Verification items for the finished model (mm, model axes). A direction names the side the tool comes from. Give positions to 0.01 mm unless a question says otherwise; leave off trailing zeros. Write each loop counter-clockwise with the first axis right and the second up, starting at its lowest first coordinate (ties: lowest second). Pieces come first, ordered by that corner, then holes. Notation, with made-up numbers: (-19, -24) - (40, -24) arc R29 cw to (40, 10) - close; hole circle Ø8 at (67.25, 19.25). An arc over 180 degrees is marked (long way). Answer as a JSON object with one key per item and string values. Group by question number.
Item 1: Go/stop test with flat-tipped pins: pin 1 (12 mm diameter, centred on x = -45, y = -17, fed in from +Z); pin 2 (6 mm diameter, centred on x = -51, y = -14.5, fed in from -Z). Record where each tip stops, or that it passes through.
Item 2: Scan lines: line 1 along X through (y, z) = (-7.5, 26); line 2 along Z through (x, y) = (-38, -12.75); line 3 along Z through (x, y) = (-54.5, -3.75). Record each from-to range of solid material in increasing order. Write a range as [from, to].
Item 3: Draft check along X on faces 4 (the face through (-61.296, -13, 18)), 5 (the face through (-43, -13, 0)), 6 (the face through (-48.884, -13, 27)). Enter one of: +X half, -X half, draft (parallel to the pull), parting line (faces both ways), or undercut.
Item 4: Sectioned sample at B-B, the plane y = -15.75. Record the boundary of the cut face in (x, z).
Item 5: Sectioned sample at A-A, the plane z = 20. Record the boundary of the cut face in (x, y).
Item 6: Tool access check on faces 1 (the face through (-37.809, -13, 27)), 2 (the face through (-55, -13, 34.945)), 3 (the face through (-43, 0, 18)). Record the directions out of +Z, -Z, +X, -X, +Y, -Y that give a thin tool (end or side, any length) a straight path to the whole face; none if there is none.
```python
from build123d import *

# Parameters (mm, degrees)
F1_DEPTH = 25.4
F4_DEPTH = 25.4


with BuildPart() as f1:
    # F0 (on Front) → F1 (new body)
    with BuildSketch(Plane.XZ):
        Polygon((-51.1758476496, 56.7135326564), (-63.5878965259, 56.522578001), (-63.5878965259, 0), (-8.4020039067, 0), (-8.4020039067, 56.522578001), (-21.959785372, 56.522578001), (-21.959785372, 11.6482349113), (-51.1758476496, 11.6482349113), align=None)
    extrude(amount=F1_DEPTH)


with BuildPart() as f4:
    # F3 (on Front) → F4 (new body)
    with BuildSketch(Plane.XZ):
        Polygon((-61.2964443862, 34.9447019398), (-61.2964443862, 33.4170646966), (-61.2964443862, 0), (-24.4421958923, 0), (-24.4421958923, 35.1356565952), (-37.809021771, 35.1356565952), (-37.809021771, 19.2864201963), (-48.8843917847, 19.2864201963), (-48.8843917847, 34.9447019398), align=None)
    extrude(amount=F4_DEPTH)


solid = f4.part
```
Geometry check:
{
 "1": {"pin 1": "z = 34.94", "pin 2": "z = 0"},
 "2": {"line 1": "[-61.3, -48.88], [-37.81, -24.44]", "line 2": "[0, 19.29]", "line 3": "[0, 34.94]"},
 "3": {"face 4": "-X half", "face 5": "draft", "face 6": "undercut"},
 "4": {"outline": "(-61.3, 0) - (-24.44, 0) - (-24.44, 35.14) - (-37.81, 35.14) - (-37.81, 19.29) - (-48.88, 19.29) - (-48.88, 34.94) - (-61.3, 34.94) - close"},
 "5": {"outline": "(-61.3, -25.4) - (-48.88, -25.4) - (-48.88, 0) - (-61.3, 0) - close; (-37.81, -25.4) - (-24.44, -25.4) - (-24.44, 0) - (-37.81, 0) - close"},
 "6": {"face 1": "+Z, +Y, -Y", "face 2": "+Z, -X, +Y, -Y", "face 3": "+Z, -Z, +X, -X, +Y"}
}
